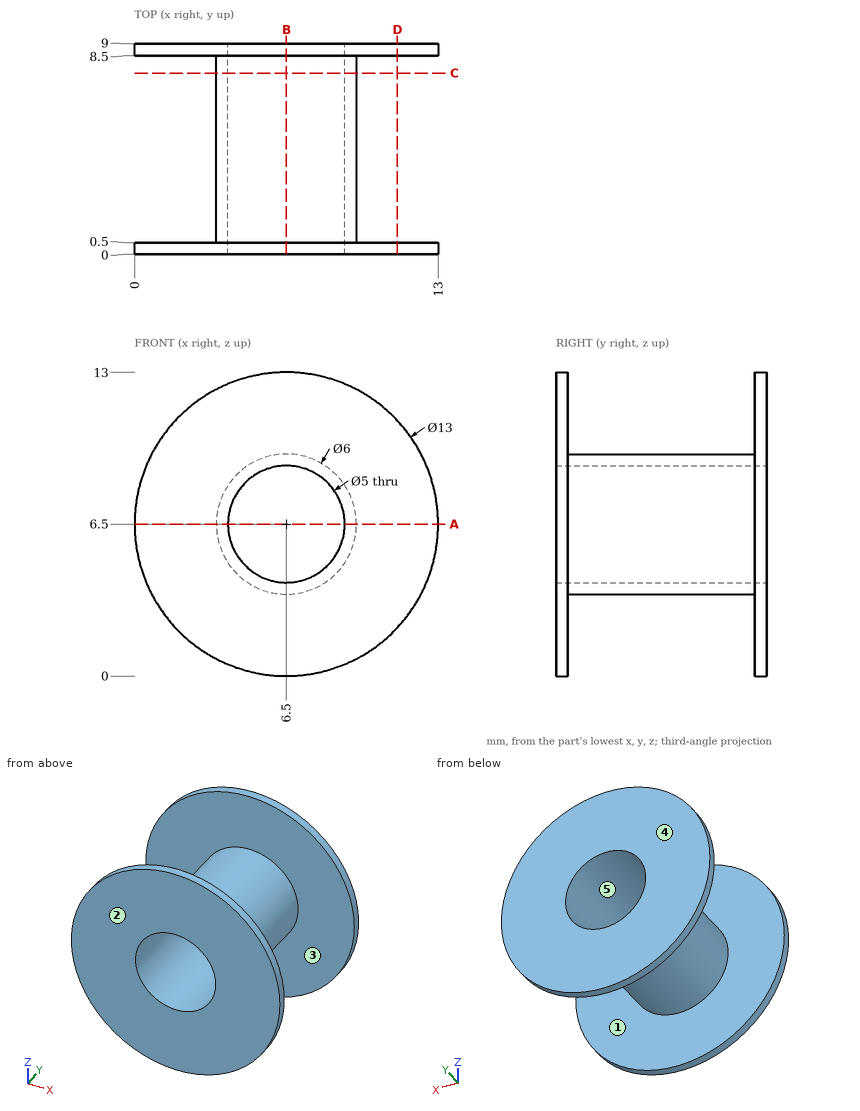
Study the drawing (mm; zero at the part's minimum x, y, z) and answer. A direction names the side the tool comes from. Round coordinates to 2 decimals unless told otherwise and drop trailing zeros. Write each loop counter-clockwise with the first axis right and the second up, starting at its lowest first coordinate (ties: lowest second). Pieces come first, ordered by that corner, then holes. Notation, with made-up numbers: (22, 78.25) -> (39, 78.25) arc R27 ccw to (39, 97.25) -> close; hole circle Ø4 at (68.5, 37). An arc over 180 degrees is marked (long way). Answer as CSV lines item,"result". Start each with the question number.
(1) The part is cut by section B-B, the plane x = 6.5. Give the vertices of the cut face in (y, z).
(2) The mould has two halves that part along Y. Classify the marked faces 3, 4 and 5: +Y half, -Y half, draft (parallel to the pull), parting line (faces both ways), or undercut.
(3) The part is cut by section D-D, the plane x = 11.25. Give the vertices of the cut face in (y, z), then the cut area to 3 significant figures.
(4) Find the intervals of material crossed by probe 1 along Y at (x, z) = (3.5, 9.75); probe 2 along Z at (x, y) = (6.5, 4.75); probe 3 along X at (y, z) = (7, 5.75), in increasing order.
(5) A tool of negligible diameter and unlimited length cuts with its end or side. For the marked faces 1 and 2, from which of +Z, -Z, +X, -X, +Y, -Y can it reach the whole face along a straight path? Write none if from no direction.
(6) The part is cut by section C-C, the plane y = 7.75. Give the vertices of the cut face in (x, z), then the cut area to 3 significant figures.
(7) The part is cut by section A-A, the plane z = 6.5. Give the vertices of the cut face in (x, y).
(8) Each of these flat-tipped pins is pushed along its axis until it touches: pin 1 (3 mm diameter, centred on x = 3.5, y = 1.5, fed in from -Z); pin 2 (2 mm diameter, centred on x = 6, y = 2, fed in from -Z); pin 3 (2 mm diameter, centred on y = 3, z = 11.5, fed in from +X); pin 4 (2 mm diameter, centred on y = 3.5, z = 9, fed in from +X). Where does it stop, or does it pass through?
Output values:
1,outline,"(0, 0) -> (0.5, 0) -> (0.5, 3.5) -> (8.5, 3.5) -> (8.5, 0) -> (9, 0) -> (9, 4) -> (0, 4) -> close; (0, 9) -> (9, 9) -> (9, 13) -> (8.5, 13) -> (8.5, 9.5) -> (0.5, 9.5) -> (0.5, 13) -> (0, 13) -> close"
2,face 3,"undercut"
2,face 4,"+Y half"
2,face 5,"draft"
3,outline,"(0, 2.06) -> (0.5, 2.06) -> (0.5, 10.94) -> (0, 10.94) -> close; (8.5, 2.06) -> (9, 2.06) -> (9, 10.94) -> (8.5, 10.94) -> close"
3,area,"8.87 mm²"
4,probe 1,"y = 0 to 0.5, 8.5 to 9"
4,probe 2,"z = 3.5 to 4, 9 to 9.5"
4,probe 3,"x = 3.6 to 4.12, 8.88 to 9.4"
5,face 1,"none"
5,face 2,"+Z, -Z, +X, -X, -Y"
6,outline,"circle Ø6 at (6.5, 6.5); hole circle Ø5 at (6.5, 6.5)"
6,area,"8.64 mm²"
7,outline,"(0, 0) -> (4, 0) -> (4, 9) -> (0, 9) -> (0, 8.5) -> (3.5, 8.5) -> (3.5, 0.5) -> (0, 0.5) -> close; (9, 0) -> (13, 0) -> (13, 0.5) -> (9.5, 0.5) -> (9.5, 8.5) -> (13, 8.5) -> (13, 9) -> (9, 9) -> close"
8,pin 1,"stops at z = 0.28"
8,pin 2,"stops at z = 3.5"
8,pin 3,"passes through"
8,pin 4,"stops at x = 9.1"
